```python
from build123d import *

# Parameters (mm, degrees)
SKETCH014_W     = 15
SKETCH014_H     = 5
PAD006_DEPTH    = 10
SKETCH015_W     = 13
SKETCH015_H     = 3
POCKET011_DEPTH = 6
SKETCH016_W     = 8
SKETCH016_H     = 1
POCKET012_DEPTH = 4.5
SKETCH017_W     = 1.48
SKETCH017_H     = 4.49
POCKET014_DEPTH = 2


with BuildPart() as part:
    # Sketch014 → Pad006 (new body)
    with BuildSketch(Plane.YZ):
        with Locations((0, 2.5)):
            Rectangle(SKETCH014_W, SKETCH014_H)
    extrude(amount=PAD006_DEPTH)

    # Sketch015 (on Face6 of Pad006) → Pocket011 (cut)
    with BuildSketch(Plane.YZ.offset(10)):
        with Locations((0, 2.5)):
            Rectangle(SKETCH015_W, SKETCH015_H)
    extrude(amount=-POCKET011_DEPTH, mode=Mode.SUBTRACT)

    # Sketch016 (on Face5 of Pocket011) → Pocket012 (cut)
    with BuildSketch(Plane.YZ.offset(10)):
        with Locations((0, 4.5)):
            Rectangle(SKETCH016_W, SKETCH016_H)
    extrude(amount=-POCKET012_DEPTH, mode=Mode.SUBTRACT)

    # Sketch017 (on Face6 of Pocket012) → Pocket014 (cut)
    with BuildSketch(Plane(origin=(0, 0, 5), x_dir=(0, -1, 0), z_dir=(0, 0, 1))):
        with Locations((-5.75, 6.745)):
            Rectangle(SKETCH017_W, SKETCH017_H)
        with Locations((5.75, 6.745)):
            Rectangle(SKETCH017_W, SKETCH017_H)
    extrude(amount=-POCKET014_DEPTH, mode=Mode.SUBTRACT)


solid = part.part
```
Part model, mm, in its own coordinate system. A direction names the side the tool comes from. Give positions to 0.01 mm unless a question says otherwise; leave off trailing zeros. Order: outer loops, then holes, each group sorted by start corner. A loop starts at its lowest first (then second) coordinate and runs counter-clockwise, first axis right, second up. Notation, with made-up numbers: M 10,30 L 16,30 A21 ccw 16,37 Z; hole C 24,75 d4. An arc over 180 degrees is marked long. Use a Markdown table: item, result. Add a question column.
(1) Saw through at A-A, the plane x = 7.5. Give the number of separate pieces and of enclosed holes in the cut face, and give its area (3 significant figures).
(2) Mould opens along Z. For faces 1 (the face through (7.8, 4, 4.5)), 2 (the face through (7, 6.5, 2)), 3 (the face through (5, 0, 0)), 4 (the face through (7, 0, 1)) say: +Z half, -Z half, draft (parallel to the pull), parting line (faces both ways), or undercut.
(3) Saw through at B-B, the plane y = 5.5. Give the cut face in (x, z).
(4) Saw through at D-D, the plane z = 4.3. Give the cut face in (x, y).
(5) 3-axis set-ups, long thin cutter, end or side, ignore diameter. For faces 5 (the face through (0, 0, 3)), 6 (the face through (5, 0, 4)), 7 (the face through (7.8, -4, 4.5)), 8 (the face through (6.7, 5.01, 4.5)): which of +Z, -Z, +X, -X, +Y, -Y reach the whole face in a straight line?
(6) Probe line 1 along Y through (x, z) = (8.5, 4.55); line 2 along Y through (x, z) = (9.5, 4.25); line 3 along Y through (x, z) = (6.5, 2.75). List the from-to ranges inside material, lowest first. Write a range as [from, to].
(7) Drop flat-ended pins along their axis: P1, Ø3, axis at y = -1.5, z = 3, coming from the -X side; P2, Ø2.5, axis at y = -1, z = 2.5, coming from the +X side. Give the stop position or say it passes through.
Answer key:
| question | item | result |
|---|---|---|
| 1 | separate pieces | 3 |
| 1 | enclosed holes | 0 |
| 1 | area | 25.0 mm^2 |
| 2 | face 1 | draft |
| 2 | face 2 | undercut |
| 2 | face 3 | -Z half |
| 2 | face 4 | undercut |
| 3 | outline | M 0,0 L 10,0 L 10,1 L 4,1 L 4,4 L 4.5,4 L 4.5,5 L 0,5 Z; M 8.99,4 L 10,4 L 10,5 L 8.99,5 Z |
| 4 | outline | M 0,-7.5 L 10,-7.5 L 10,-4 L 5.5,-4 L 5.5,4 L 10,4 L 10,7.5 L 0,7.5 Z; hole M 4.5,-6.49 L 8.99,-6.49 L 8.99,-5.01 L 4.5,-5.01 Z; hole M 4.5,5.01 L 8.99,5.01 L 8.99,6.49 L 4.5,6.49 Z |
| 5 | face 5 | +Z, -Z, -X, +Y, -Y |
| 5 | face 6 | +X |
| 5 | face 7 | +Z, +X |
| 5 | face 8 | +Z |
| 6 | line 1 | [-7.5, -6.49], [-5.01, -4], [4, 5.01], [6.49, 7.5] |
| 6 | line 2 | [-7.5, -4], [4, 7.5] |
| 6 | line 3 | [-7.5, -6.5], [6.5, 7.5] |
| 7 | P1 | x = 0 |
| 7 | P2 | x = 4 |
